Source: three-view drawing plus pictorial views. Frame: mm from the lowest corner of the part. A direction names the side the tool comes from. Round coordinates to 2 decimals unless told otherwise and drop trailing zeros. Loops run counter-clockwise (first coordinate to the right, second up) from the corner with the lowest first, then second, coordinate; pieces in that order, holes last. Notation, with made-up numbers: M 1,39 L 33,39 A31 ccw 33,76 Z; hole C 88.25,36.5 d4. An arc over 180 degrees is marked long. Return JSON: item names as keys, results as strings. Group by question number.
1) Access query for the marked faces 4 and 5. Directions: +Z, -Z, +X, -X, +Y, -Y. A direction counts if a zero-diameter tool reaches every point of the face in a straight line with its end or side. Return the directions, or none.
2) Section B-B (y = 2.75). Count the separate pieces of the cut face and the enclosed holes in it, plus the area to 3 significant figures.
3) Material intervals for line 1 (X direction, y = 0.5, z = 27.5) (1 decimal); line 2 (Z direction, x = 26, y = 1.75); line 3 (Z direction, x = 40, y = 5) (1 decimal), sorted ascending. Write a range as from..to.
4) Contact query for a flat-ended pin moving along its axis: P1, Ø2.5, axis at y = 4.5, z = 59.5, coming from the +X side. Output: stop coordinate, or through.
5) Mould query, pull axis Z, two halves, no side actions, for the marked faces 1, 2 and 3. Classes: +Z half, -Z half, draft (parallel to the pull), parting line (faces both ways), or undercut.
6) Section D-D (z = 12). Output: boundary loops of the cut face in (x, y).
7) Section A-A (z = 25.4). Output: boundary loops of the cut face in (x, y) (1 decimal).
8) Section C-C (x = 6.5). Output: boundary loops of the cut face in (y, z).
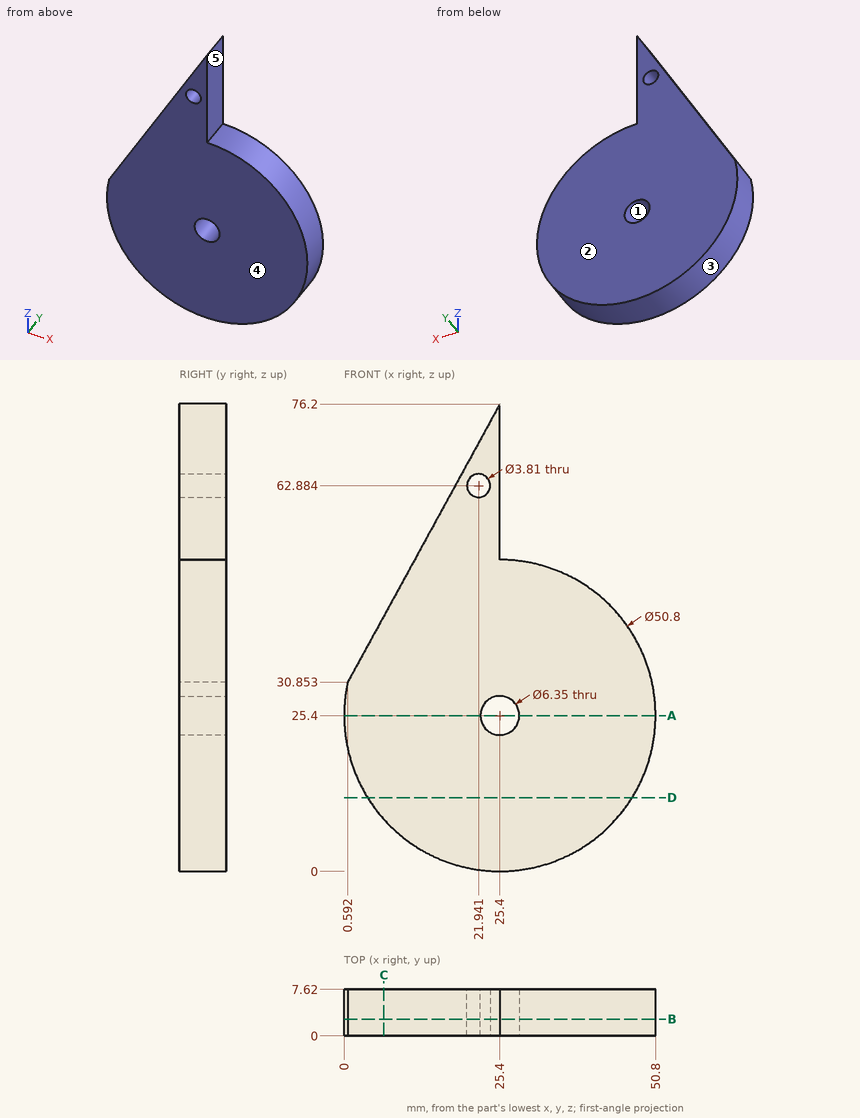
Returned:
{
 "1": {"face 4": "+Z, -Z, +X, -X, -Y", "face 5": "+Z, +X, +Y, -Y"},
 "2": {"separate pieces": "1", "enclosed holes": "2", "area": "2,180 mm^2"},
 "3": {"line 1": "x = 0.1..23, 27.8..50.7", "line 2": "z = 0.01..22.28, 28.52..50.79", "line 3": "z = 4.6..46.2"},
 "4": {"P1": "stops at x = 25.4"},
 "5": {"face 1": "undercut", "face 2": "draft", "face 3": "parting line"},
 "6": {"outline": "M 3.82,0 L 46.98,0 L 46.98,7.62 L 3.82,7.62 Z"},
 "7": {"outline": "M 0,0 L 22.2,0 L 22.2,7.6 L 0,7.6 Z; M 28.6,0 L 50.8,0 L 50.8,7.6 L 28.6,7.6 Z"},
 "8": {"outline": "M 0,8.43 L 7.62,8.43 L 7.62,41.65 L 0,41.65 Z"}
}
